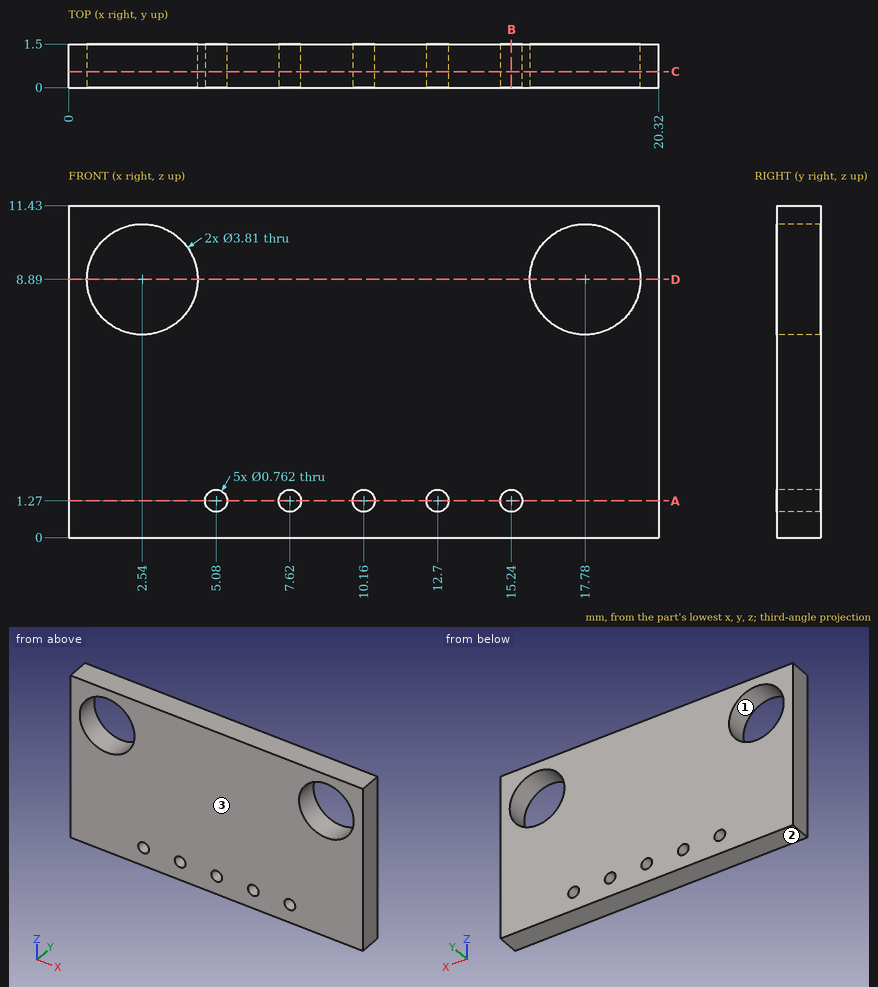
Can you work these out from the drawing? Everything is in mm from the part's minimum corner. Give positions to 0.01 mm unless a question says otherwise; leave off trailing zeros. Order: outer loops, then holes, each group sorted by start corner. A loop starts at its lowest first (then second) coordinate and runs counter-clockwise, first axis right, second up.
1. Suppose I cut it at C-C (y = 0.55). List the corners of the cut face in (x, z) for me (3 decimals).
2. We'd pull the mould along Z, two halves only. Please class the marked faces 1, 2 and 3: pulls with the +Z half, pulls with the -Z half, needs draft (parallel to the pull), parting line crosses it, or undercut.
3. I need wall thicknesses on L1, parallel to X at y = 0.7, z = 8.75; L2, parallel to X at y = 0.5, z = 1.27; L3, parallel to Z at x = 15.25, y = 1.1. Which ranges of each line are inside material? Lowest first, please.
4. Suppose I cut it at A-A (z = 1.27). List the corners of the cut face in (x, y) for me, plus the area to 3 significant figures.
5. Suppose I cut it at B-B (x = 15.24). List the corners of the cut face in (y, z) for me.
6. Suppose I cut it at D-D (z = 8.89). List the corners of the cut face in (x, y) for me (3 decimals).
7. Will this pin go through, and if not, where does the flat tip stop? P1, Ø1.5, axis at x = 17.5, z = 8, coming from the -Y side.
Solved:
1. outline: (0, 0) - (20.32, 0) - (20.32, 11.43) - (0, 11.43) - close; hole circle Ø3.81 at (2.54, 8.89); hole circle Ø0.762 at (5.08, 1.27); hole circle Ø0.762 at (7.62, 1.27); hole circle Ø0.762 at (10.16, 1.27); hole circle Ø0.762 at (12.7, 1.27); hole circle Ø0.762 at (15.24, 1.27); hole circle Ø3.81 at (17.78, 8.89)
2. face 1: undercut
2. face 2: pulls with the -Z half
2. face 3: needs draft
3. L1: x = 0 to 0.64, 4.44 to 15.88, 19.68 to 20.32
3. L2: x = 0 to 4.7, 5.46 to 7.24, 8 to 9.78, 10.54 to 12.32, 13.08 to 14.86, 15.62 to 20.32
3. L3: z = 0 to 0.89, 1.65 to 11.43
4. outline: (0, 0) - (4.7, 0) - (4.7, 1.5) - (0, 1.5) - close; (5.46, 0) - (7.24, 0) - (7.24, 1.5) - (5.46, 1.5) - close; (8, 0) - (9.78, 0) - (9.78, 1.5) - (8, 1.5) - close; (10.54, 0) - (12.32, 0) - (12.32, 1.5) - (10.54, 1.5) - close; (13.08, 0) - (14.86, 0) - (14.86, 1.5) - (13.08, 1.5) - close; (15.62, 0) - (20.32, 0) - (20.32, 1.5) - (15.62, 1.5) - close
4. area: 24.8 mm2
5. outline: (0, 0) - (1.5, 0) - (1.5, 0.89) - (0, 0.89) - close; (0, 1.65) - (1.5, 1.65) - (1.5, 11.43) - (0, 11.43) - close
6. outline: (0, 0) - (0.635, 0) - (0.635, 1.5) - (0, 1.5) - close; (4.445, 0) - (15.875, 0) - (15.875, 1.5) - (4.445, 1.5) - close; (19.685, 0) - (20.32, 0) - (20.32, 1.5) - (19.685, 1.5) - close
7. P1: passes through
